Design review of the part built by this model. Coordinates are the model's own, in mm. A direction names the side the tool comes from. Coordinates: 2 decimals unless noted, no trailing zeros. Write each loop counter-clockwise with the first axis right and the second up, starting at its lowest first coordinate (ties: lowest second). Pieces come first, ordered by that corner, then holes. Notation, with made-up numbers: (-27.5, -12.5) - (14.5, -12.5) arc R20 cw to (14.5, 11.5) - close; hole circle Ø2 at (-23, 87.25). An arc over 180 degrees is marked (long way). Answer as a JSON object with one key per item and string values.
```python
from build123d import *

# Parameters (mm, degrees)
SKETCH1_R           = 40
BOSS_EXTRUDE1_DEPTH = 30
SKETCH2_R           = 5
BOSS_EXTRUDE2_DEPTH = 30
CIRPATTERN1_COUNT   = 4


with BuildPart() as part:
    # Sketch1 → Boss-Extrude1 (new body)
    with BuildSketch(Plane(origin=(0, 0, 0), x_dir=(1, 0, 0), z_dir=(0, 1, 0))):
        Polygon((11.5, 125), (-11.5, 125), (-54.518512439, 54.518512439), (-125, 11.5), (-125, -11.5), (-54.518512439, -54.518512439), (-11.5, -125), (11.5, -125), (54.518512439, -54.518512439), (125, -11.5), (125, 11.5), (54.518512439, 54.518512439), align=None)
        with Locations(Location((0, 0, 0), (0, 0, 270))):
            Circle(SKETCH1_R, mode=Mode.SUBTRACT)
    extrude(amount=BOSS_EXTRUDE1_DEPTH)

    # Sketch2 → Boss-Extrude2 (add)
    with BuildSketch(Plane.XY.offset(125)):
        with Locations((0, 15)):
            Circle(SKETCH2_R)
    boss_extrude2 = extrude(amount=BOSS_EXTRUDE2_DEPTH)

    # CirPattern1: Boss-Extrude2 ×4 about axis
    cirpattern1_axis = Axis((0, 0, 0), (0, 1, 0))
    for i in range(1, CIRPATTERN1_COUNT):
        add(boss_extrude2.rotate(cirpattern1_axis, i * 360 / CIRPATTERN1_COUNT))


solid = part.part
```
(1) Tool access review of faces 1 (the face through (1.08, 10.12, -139.79)), 2 (the face through (33.31, 14.79, -89.27)): name each direction out of +Z, -Z, +X, -X, +Y, -Y from which nothing blocks a thin tool from reaching the whole face with its end or side.
Solved:
{"face 1": "-Z", "face 2": "-Z, +X, +Y, -Y"}
(2) Take a section at C-C, the plane x = 34.5. Write out the cut boundary in (y, z).
Solved:
{"outline": "(0, -87.32) - (30, -87.32) - (30, -20.24) - (0, -20.24) - close; (0, 20.24) - (30, 20.24) - (30, 87.32) - (0, 87.32) - close"}
(3) For pin 1 (8 mm diameter, centred on y = 16, z = -119.5, fed in from -X); pin 2 (12 mm diameter, centred on y = 11, z = 41.5, fed in from +X); pin 3 (10 mm diameter, centred on x = 72.5, y = 6, fed in from +Z), all flat-tipped, find the tip position at first contact; note any pin that passes through.
Solved:
{"pin 1": "stops at x = -17.3", "pin 2": "stops at x = 85.68", "pin 3": "stops at z = 46.6"}
(4) To check wall thickness, follow line 1 (X direction, y = 7.25, z = 0); line 2 (X direction, y = 18.5, z = 0); line 3 (Z direction, x = -2, y = 3). State the ranges of each line that lie inside material, in increasing order. Write a range as from..to.
Solved:
{"line 1": "x = -125..-40, 40..125", "line 2": "x = -155..-40, 40..155", "line 3": "z = -125..-39.95, 39.95..125"}
(5) Take a section at D-D, the plane x = -26.5. Write out the cut boundary in (y, z).
Solved:
{"outline": "(0, -100.42) - (30, -100.42) - (30, -29.96) - (0, -29.96) - close; (0, 29.96) - (30, 29.96) - (30, 100.42) - (0, 100.42) - close"}
(6) Take a section at B-B, the plane z = 0. Write out the cut boundary in (x, y), and give its area (3 significant figures).
Solved:
{"outline": "(-155, 10) - (-125, 10) - (-125, 0) - (-40, 0) - (-40, 30) - (-125, 30) - (-125, 20) - (-155, 20) - close; (40, 0) - (125, 0) - (125, 10) - (155, 10) - (155, 20) - (125, 20) - (125, 30) - (40, 30) - close", "area": "5,700 mm^2"}
